For this review, take the finished solid that the model builds, in its own axes (mm). Face numbers are marked on the shaded views. A direction names the side the tool comes from. Give positions to 0.01 mm unless a question says otherwise; leave off trailing zeros. Write each loop counter-clockwise with the first axis right and the second up, starting at its lowest first coordinate (ties: lowest second). Pieces come first, ordered by that corner, then holes.
Q1. Insertion check: P1, Ø1, axis at x = -3.5, y = 4, coming from the +Z side; P2, Ø2, axis at y = 5.5, z = 1, coming from the -X side; P3, Ø1.5, axis at y = -5.5, z = 3, coming from the -X side. Each pin has a flat end and moves straight along its axis. Give the tip position at first contact, or say it passes through.
Q2. We need section C-C (z = 0.7). Write out the cut boundary in (x, y), then the cut area to 3 significant figures.
Q3. Machinability: for the marked faces 1 and 2, which of the approach directions +Z, -Z, +X, -X, +Y, -Y give a long, thin tool a straight path to every point of the face, cutting with its end or side? Answer none if there is none.
Q4. We need section A-A (x = 0). Write out the cut boundary in (y, z).
Q5. We need section D-D (y = 4). Give the number of separate pieces and of enclosed holes in the cut face, then the cut area to 3 significant figures.
Q6. We need section B-B (y = -6.25). Write out the cut boundary in (x, z).
Q7. Mouldability with a two-part tool opening along X and no side actions: class the marked faces 3, 4 and 5 as released by +X, released by -X, zero draft, split by the parting line, or undercut.
Q8. For line 1 (X direction, y = 1.75, z = 1.35); line 2 (Y direction, x = 0, z = 2.95); line 3 (X direction, y = 0.75, z = 4.1), list the stretches that pass through material, from the lowest coordinate up.
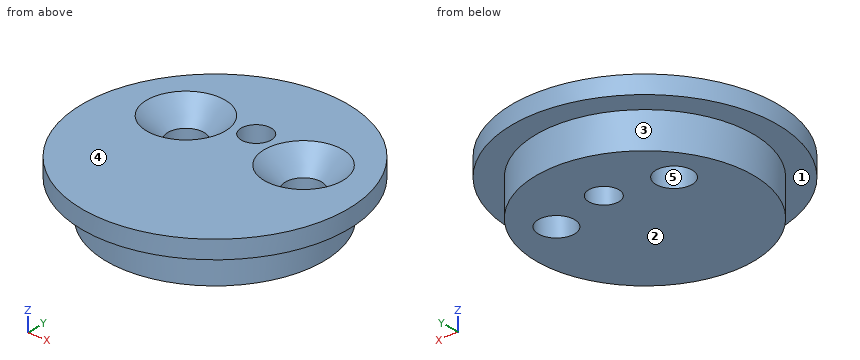
Autodesk Inventor part; units mm, degrees
ref_plane "YZ Plane" through (0, 0, 0) normal (1, 0, 0) x (0, 1, 0)
ref_plane "XZ Plane" through (0, 0, 0) normal (0, 1, 0) x (-1, 0, 0)
ref_plane "XY Plane" through (0, 0, 0) normal (0, 0, 1) x (1, 0, 0)
sketch "スケッチ1" plane through (0, 0, 0) normal (0, 0, 1) x (1, 0, 0)
  circle A0 centre (0, 0) radius 9
  line L0 (-5, 2.8868) -> (5, 2.8868) construction
  line L1 (5, 2.8868) -> (0, -5.7735) construction
  line L2 (0, -5.7735) -> (-5, 2.8868) construction
  circle A1 centre (-5, 2.8868) radius 1.5
  circle A2 centre (5, 2.8868) radius 1.5
  circle A3 centre (0, -5.7735) radius 1.5
  circle A4 centre (0, 4) radius 1.25
  line L3 (0, 0) -> (0, 4) construction
  circle A5 centre (0, 0) radius 10
  dimension "d0" = 18
  dimension "d1" = 10
  dimension "d2" = 3
  dimension "d3" = 3
  dimension "d4" = 3
  dimension "d5" = 2.5
  dimension "d6" = 4
  dimension "d12" = 1
extrude "押し出し1" add sketch "スケッチ1" along normal blind 4.5 contours A0 | A3
sketch "スケッチ2" plane through (0, 0, 4.5) normal (0, 0, 1) x (1, 0, 0)
  circle A0 centre (0, 0) radius 11
  circle A1 centre (5, 2.8868) radius 1.5
  circle A2 centre (-5, 2.8868) radius 1.5
  circle A3 centre (0, 4) radius 1.25
  circle A4 centre (0, 0) radius 9
  dimension "d15" = 2
extrude "押し出し2" add sketch "スケッチ2" against normal blind 1.5 contours A0
chamfer "面取り2" distance 1.75 angle 45 2 edges at (-6.5, 2.8868, 4.5) (3.5, 2.8868, 4.5)
properties part number "横回転最終段カム" material "アルミニウム 2014-T4"
Computed:
1. P1: stops at z = 3.62
1. P2: stops at x = -7.79
1. P3: stops at x = -9.92
2. outline: circle Ø18 at (0, 0); hole circle Ø3 at (-5, 2.89); hole circle Ø2.5 at (0, 4); hole circle Ø3 at (5, 2.89)
2. area: 235 mm2
3. face 1: -Z
3. face 2: -Z, +X, -X, +Y, -Y
4. outline: (-11, 3) - (-9, 3) - (-9, 0) - (2.75, 0) - (2.75, 4.5) - (-11, 4.5) - close; (5.25, 0) - (9, 0) - (9, 3) - (11, 3) - (11, 4.5) - (5.25, 4.5) - close
5. separate pieces: 4
5. enclosed holes: 0
5. area: 42.3 mm2
6. outline: (-9.05, 3) - (-6.48, 3) - (-6.48, 0) - (6.48, 0) - (6.48, 3) - (9.05, 3) - (9.05, 4.5) - (-9.05, 4.5) - close
7. face 3: split by the parting line
7. face 4: zero draft
7. face 5: undercut
8. line 1: x = -8.83 to -5.98, -4.02 to 4.02, 5.98 to 8.83
8. line 2: y = -9 to 2.75, 5.25 to 9
8. line 3: x = -10.97 to -6.89, -3.11 to 3.11, 6.89 to 10.97
